Can you work these out from the model? Positions are in its coordinate system, mm. A direction names the side the tool comes from. Coordinates: 2 decimals unless noted, no trailing zeros. Order: outer loops, then holes, each group sorted by start corner. A loop starts at its lowest first (then second) coordinate and runs counter-clockwise, first axis right, second up. Notation, with made-up numbers: (-23.75, -32.5) -> (-11.75, -32.5) arc R21 ccw to (-11.75, -9.5) -> close; hole circle Ø3 at (34, 44.25). An arc over 180 degrees is marked (long way). Write item = value, one per line.
```python
from build123d import *

# Parameters (mm, degrees)
F0_W     = 0.0285906434
F0_H     = 5
F0_W_2   = 41.8
F0_R     = 1.8
F1_DEPTH = 2.5
F2_R     = 2.5
F3_SIZE  = 0.75


# Not quite as in the source:
# - a feature names something its author has since deleted; it is built from what else it names


with BuildPart() as f1:
    # F0 (on Front) → F1 (new body)
    with BuildSketch(Plane.XZ):
        with Locations((-41.8142953217, 18.525)):
            Rectangle(F0_W, F0_H)
        with Locations((41.8142953217, 18.525)):
            Rectangle(F0_W, F0_H)
        with Locations((-20.9, 18.525)):
            Rectangle(F0_W_2, F0_H)
        with Locations((20.9, 18.525)):
            Rectangle(F0_W_2, F0_H)
        with Locations((20.9, 42.125)):
            Rectangle(F0_W_2, F0_H)
        Polygon((41.8, 64.625), (41.8, 44.625), (41.8, 39.625), (41.8, 21.025), (41.8285906434, 21.025), (41.8285906434, 16.025), (41.8, 16.025), (41.8, -3.975), (50.4, -3.975), (50.4, 64.625), align=None)
        with Locations((46.1, 0.325)):
            Circle(F0_R, mode=Mode.SUBTRACT)
        with Locations((46.1, 48.525)):
            Circle(F0_R, mode=Mode.SUBTRACT)
        with Locations((46.1, 60.325)):
            Circle(F0_R, mode=Mode.SUBTRACT)
        with Locations((-20.9, 42.125)):
            Rectangle(F0_W_2, F0_H)
        Polygon((-41.8, 64.625), (-50.4, 64.625), (-50.4, -3.975), (-41.8, -3.975), (-41.8, 16.025), (-41.8285906434, 16.025), (-41.8285906434, 21.025), (-41.8, 21.025), (-41.8, 39.625), (-41.8, 44.625), align=None)
        with Locations((-46.1, 0.325)):
            Circle(F0_R, mode=Mode.SUBTRACT)
        with Locations((-46.1, 48.525)):
            Circle(F0_R, mode=Mode.SUBTRACT)
        with Locations((-46.1, 60.325)):
            Circle(F0_R, mode=Mode.SUBTRACT)
    extrude(amount=F1_DEPTH)

    # F2
    f2_edges = [f1.edges().sort_by_distance(p)[0] for p in [
        (-41.8, -1.25, 44.625),
        (41.8, -1.25, 44.625),
        (-41.8, -1.25, 39.625),
        (41.8, -1.25, 39.625),
        (-41.8, -1.25, 21.025),
        (41.8, -1.25, 21.025),
        (-41.8, -1.25, 16.025),
        (41.8, -1.25, 16.025),
        (41.8, -1.25, -3.975),
        (50.4, -1.25, -3.975),
        (-50.4, -1.25, -3.975),
        (-41.8, -1.25, -3.975),
        (50.4, -1.25, 64.625),
        (41.8, -1.25, 64.625),
        (-50.4, -1.25, 64.625),
        (-41.8, -1.25, 64.625),
    ]]
    fillet(f2_edges, radius=F2_R)

    # F3
    f3_edges = [f1.edges().sort_by_distance(p)[0] for p in [
        (0, 0, 16.025),
        (0, 0, 39.625),
        (-46.1, -2.5, 64.625),
        (0, -2.5, 39.625),
    ]]
    chamfer(f3_edges, length=F3_SIZE)


solid = f1.part
```
Item 1: For faces 1 (the conical face through (-41.19, -1.953, 45.193)), 2 (the conical face through (41.2, -0.54, 15.46)), 3 (the conical face through (-41.232, -1.953, 15.415)), which set-ups out of +Z, -Z, +X, -X, +Y, -Y let a thin tool reach every point of the face, with its end or its side?
A:
face_1 = +Z, -Y
face_2 = -Z, +Y
face_3 = -Z, -Y
Item 2: If we mould it in two halves opening along X, with no side actions, what happens to faces 4 (the conical face through (42.837, -2.203, -2.906)), 5 (the conical face through (49.324, -0.286, -2.931)), 6 (the conical face through (-49.33, -2.2, 63.59))? For each: pulls with the +X half, pulls with the -X half, needs draft (parallel to the pull), parting line crosses it, or undercut.
A:
face_4 = undercut
face_5 = pulls with the +X half
face_6 = pulls with the -X half
Item 3: I want a section at B-B, the plane x = 46.1. Please give me the cut outline in (y, z) (3 decimals).
A:
outline = (-2.5, -3.225) -> (-1.75, -3.975) -> (-0.75, -3.975) -> (0, -3.225) -> (0, -1.475) -> (-2.5, -1.475) -> close; (-2.5, 2.125) -> (0, 2.125) -> (0, 46.725) -> (-2.5, 46.725) -> close; (-2.5, 50.325) -> (0, 50.325) -> (0, 58.525) -> (-2.5, 58.525) -> close; (-2.5, 62.125) -> (0, 62.125) -> (0, 63.875) -> (-0.75, 64.625) -> (-1.75, 64.625) -> (-2.5, 63.875) -> close
Item 4: If I drill on probe 1 along Z at (x, y) = (-46.1, -1.15) (3 decimals); probe 2 along X at (y, z) = (-1.5, 48.5); probe 3 along Z at (x, y) = (-11, -0.95) (3 decimals), over which ranges is the centre line in solid material (lowest first)?
A:
probe_1 = -3.975 to -1.475, 2.125 to 46.725, 50.325 to 58.525, 62.125 to 64.625
probe_2 = -50.4 to -47.9, -44.3 to -41.8, 41.8 to 44.3, 47.9 to 50.4
probe_3 = 16.025 to 21.025, 39.625 to 44.625
Item 5: I'm going to push flat-ended pins straight in: P1, Ø6, axis at x = -17.5, z = 11, coming from the -Y side; P2, Ø0.8, axis at x = 14, y = -1.5, coming from the -Z side (3 decimals); P3, Ø1.1, axis at x = 14, y = -1.5, coming from the +Z side (3 decimals); P4, Ø6, axis at x = 27.5, z = 47.5, coming from the +Y side (3 decimals). Where does each tip first touch, or does it pass through?
A:
P1 = through
P2 = 16.025
P3 = 44.625
P4 = -0.625
Item 6: I want a section at C-C, the plane z = 11. Please give me the cut outline in (x, y).
A:
outline = (-50.4, -1.75) -> (-49.65, -2.5) -> (-42.55, -2.5) -> (-41.8, -1.75) -> (-41.8, -0.75) -> (-42.55, 0) -> (-49.65, 0) -> (-50.4, -0.75) -> close; (41.8, -1.75) -> (42.55, -2.5) -> (49.65, -2.5) -> (50.4, -1.75) -> (50.4, -0.75) -> (49.65, 0) -> (42.55, 0) -> (41.8, -0.75) -> close
Item 7: I want a section at A-A, the plane x = 7. Please give me the cut outline in (y, z) (3 decimals), plus the area to 4 significant figures.
A:
outline = (-2.5, 16.775) -> (-1.75, 16.025) -> (-0.75, 16.025) -> (0, 16.775) -> (0, 20.275) -> (-0.75, 21.025) -> (-1.75, 21.025) -> (-2.5, 20.275) -> close; (-2.5, 40.375) -> (-1.75, 39.625) -> (-0.75, 39.625) -> (0, 40.375) -> (0, 43.875) -> (-0.75, 44.625) -> (-1.75, 44.625) -> (-2.5, 43.875) -> close
area = 22.75 mm2
